Autodesk Inventor part; units mm, degrees
ref_plane "YZ Plane" through (0, 0, 0) normal (1, 0, 0) x (0, 1, 0)
ref_plane "XZ Plane" through (0, 0, 0) normal (0, 1, 0) x (-1, 0, 0)
ref_plane "XY Plane" through (0, 0, 0) normal (0, 0, 1) x (1, 0, 0)
sketch "Sketch1" plane through (0, 0, 0) normal (0, 0, 1) x (1, 0, 0)
  circle A0 centre (0, 0) radius 9.25
  circle A1 centre (0, 0) radius 5.75
  dimension "d0" = 11.5
  dimension "d1" = 18.5
extrude "Extrusion1" add sketch "Sketch1" along normal blind 1.75
sketch "Sketch2" plane through (0, 0, 1.75) normal (0, 0, 1) x (1, 0, 0)
  circle A0 centre (0, 0) radius 5.75
  circle A1 centre (0, 7.5) radius 1.4
  dimension "d4" = 7.5
  dimension "d5" = 2.8
extrude "Extrusion2" add sketch "Sketch2" along normal blind 0.01 contours A1
pattern_circular "Circular Pattern1" count 10 over 360 about axis through (0, 0, 0) along (0, 0, 1) of "Extrusion2"
properties part number "Capsule.contactring"
Model file for the job. Use its own axes, mm. Give positions to 0.01 mm unless a question says otherwise; leave off trailing zeros. Loops run counter-clockwise (first coordinate to the right, second up) from the corner with the lowest first, then second, coordinate; pieces in that order, holes last.
1) Flat gauge pins, fed straight in: pin 1 Ø1 at (y, z) = (2.5, 1.5) entering from -X; pin 2 Ø4 at (x, y) = (-2, -0.5) entering from +Z (1 decimal). Where does each tip first touch, or does it go through?
2) Saw through at B-B (y = -4). Write the cut outline in (x, z), plus the area to 3 significant figures.
3) Saw through at C-C (z = 1.2). Write the cut outline in (x, y), plus the area to 3 significant figures.
4) Wall check: line 1 (Y direction, x = 0, z = 1.05); line 2 (X direction, y = 2.25, z = 1.35); line 3 (Z direction, x = 5, y = 4.25). Give the ranges that are in metal, low to high.
5) Pull direction Y, two halves, no side cores. Call faces 1 (the cylindrical face through (-2.01, 9.03, 0.86)), 2 (the flat face through (4, -6, 1.76)), 3 (the cylindrical face through (-0.75, -5.7, 0.86)): +Y half, -Y half, draft (parallel to the pull), parting line (faces both ways), or undercut.
Answer block:
1. pin 1: stops at x = -9.03
1. pin 2: passes through
2. outline: (-8.34, 0) - (-4.13, 0) - (-4.13, 1.75) - (-8.34, 1.75) - close; (4.13, 0) - (8.34, 0) - (8.34, 1.75) - (4.13, 1.75) - close
2. area: 14.7 mm2
3. outline: circle Ø18.5 at (0, 0); hole circle Ø11.5 at (0, 0)
3. area: 165 mm2
4. line 1: y = -9.25 to -5.75, 5.75 to 9.25
4. line 2: x = -8.97 to -5.29, 5.29 to 8.97
4. line 3: z = 0 to 1.75
5. face 1: parting line
5. face 2: draft
5. face 3: undercut
